Work out the finished part from the listing and answer in its coordinate system (mm). A direction names the side the tool comes from. Give positions to 0.01 mm unless a question says otherwise; leave off trailing zeros. Loops run counter-clockwise (first coordinate to the right, second up) from the corner with the lowest first, then second, coordinate; pieces in that order, holes last. Notation, with made-up numbers: M -17.5,81 L -7.5,81 A25 ccw -7.5,96 Z; hole C 15,31 d1. An arc over 180 degrees is marked long. Write item = value, one per line. Start each with the question number.
1. Section C-C on x = 9 is taken. Determine the outline of the cut face in (y, z).
2. Section D-D on y = 4 is taken. Give the number of separate pieces and of enclosed holes in the cut face, plus the area to 3 significant figures.
3. Flat-ended cylindrical pins translate along their axes: pin 1 Ø12 at (y, z) = (-11.5, 3.5) entering from -X; pin 2 Ø17 at (y, z) = (-7.5, 8) entering from +X; pin 3 Ø8 at (x, y) = (-22, -8.75) entering from -Z. Find the tip coordinate at first contact, or state that the pin passes through.
4. The mould has two halves that part along X. Classify faces 4 (the face through (-13, 0, 13)), 5 (the face through (10.5, -0.3, 17)), 6 (the face through (27, 15, 18)): released by +X, released by -X, zero draft, split by the parting line, or undercut.
5. Consider L1, parallel to Y at x = -22, z = 18; L2, parallel to X at y = 16, z = 14; L3, parallel to Z at x = -6, y = -16. Determine where each line is inside the solid, lowest interval first. Write a range as [from, to].
6. Section B-B on z = 7.5 is taken. Determine the outline of the cut face in (x, y).
7. For faces 1 (the face through (16, 0, -17)), 2 (the face through (48, 0, 17)), 3 (the face through (16.5, 0, -18)), determine the directions among +Z, -Z, +X, -X, +Y, -Y from which every point of the face is accessible in a straight line to the end or side of a thin tool.
8. Section A-A on x = 48.5 is taken. Determine the outline of the cut face in (y, z).
```python
from build123d import *

# Parameters (mm, degrees)
F0_W          = 24
F0_H          = 34
F1_DEPTH      = 18.75
F1_DEPTH_BACK = 18.75
F2_R          = 2.5
F3_DEPTH      = 2.5
F2_W          = 6.75
F2_H          = 30
F2_W_2        = 13.25
F4_DEPTH      = 60
F5_W          = 29.5
F5_H          = 28.5
F6_DEPTH      = 76.15809
F6_DEPTH_BACK = 25


with BuildPart() as f1:
    # F0 (on Front) → F1 (new body, two sides)
    with BuildSketch(Plane.XZ) as f1_sk:
        Polygon((14.5, 19.5), (-14.5, 19.5), (-14.5, -19.5), (14.5, -19.5), (41, -19.5), (41, -17), (41, 17), (41, 19.5), align=None)
        Rectangle(F0_W, F0_H, mode=Mode.SUBTRACT)
        with Locations((26.5, 0)):
            Rectangle(F0_W, F0_H, mode=Mode.SUBTRACT)
    extrude(amount=F1_DEPTH)
    extrude(f1_sk.sketch, amount=-F1_DEPTH_BACK)

    # F2 (on face) → F3 (join)
    with BuildSketch(Plane.XY.offset(19.5)):
        Polygon((-29.5, 18.75), (-29.5, -18.75), (56, -18.75), (56, 18.75), (-14.5, 18.75), align=None)
        with Locations((-22, -8.75)):
            Circle(F2_R, mode=Mode.SUBTRACT)
        with Locations((48.5, -8.75)):
            Circle(F2_R, mode=Mode.SUBTRACT)
        with Locations((-22, 8.75)):
            Circle(F2_R, mode=Mode.SUBTRACT)
        Polygon((-10, -15), (-10, 15), (3.25, 15), (10, 15), (16.5, 15), (23.25, 15), (36.5, 15), (36.5, -15), (23.25, -15), (16.5, -15), (10, -15), (3.25, -15), align=None, mode=Mode.SUBTRACT)
        with Locations((48.5, 8.75)):
            Circle(F2_R, mode=Mode.SUBTRACT)
    extrude(amount=-F3_DEPTH)

    # F2 (on face) → F4 (cut)
    with BuildSketch(Plane.XY.offset(19.5)):
        with Locations((6.625, 0)):
            Rectangle(F2_W, F2_H)
        with Locations((-3.375, 0)):
            Rectangle(F2_W_2, F2_H)
        with Locations((19.875, 0)):
            Rectangle(F2_W, F2_H)
        with Locations((29.875, 0)):
            Rectangle(F2_W_2, F2_H)
    extrude(amount=-F4_DEPTH, mode=Mode.SUBTRACT)

    # F5 (on Right) → F6 (cut, two sides)
    with BuildSketch(Plane.YZ) as f6_sk:
        with Locations((0, -1.25)):
            Rectangle(F5_W, F5_H)
    extrude(amount=F6_DEPTH, mode=Mode.SUBTRACT)
    extrude(f6_sk.sketch, amount=-F6_DEPTH_BACK, mode=Mode.SUBTRACT)


solid = f1.part
```
Verdict:
q1.outline = M -18.75,-19.5 L -15,-19.5 L -15,-17 L -18.75,-17 Z; M -18.75,17 L -15,17 L -15,19.5 L -18.75,19.5 Z; M 15,-19.5 L 18.75,-19.5 L 18.75,-17 L 15,-17 Z; M 15,17 L 18.75,17 L 18.75,19.5 L 15,19.5 Z
q2.separate_pieces = 6
q2.enclosed_holes = 0
q2.area = 194 mm2
q3.pin_1 = -14.5
q3.pin_2 = 41
q3.pin_3 = 17
q4.face_4 = zero draft
q4.face_5 = undercut
q4.face_6 = undercut
q5.L1 = [-18.75, -11.25], [-6.25, 6.25], [11.25, 18.75]
q5.L2 = [-14.5, -12], [12, 14.5], [38.5, 41]
q5.L3 = [-19.5, -17], [17, 19.5]
q6.outline = M -14.5,-18.75 L -12,-18.75 L -12,-14.75 L -14.5,-14.75 Z; M -14.5,14.75 L -12,14.75 L -12,18.75 L -14.5,18.75 Z; M 12,-18.75 L 14.5,-18.75 L 14.5,-14.75 L 12,-14.75 Z; M 12,14.75 L 14.5,14.75 L 14.5,18.75 L 12,18.75 Z; M 38.5,-18.75 L 41,-18.75 L 41,-14.75 L 38.5,-14.75 Z; M 38.5,14.75 L 41,14.75 L 41,18.75 L 38.5,18.75 Z
q7.face_1 = +Y, -Y
q7.face_2 = -Z, +X, +Y, -Y
q7.face_3 = +Z, -Z
q8.outline = M -18.75,17 L -11.25,17 L -11.25,19.5 L -18.75,19.5 Z; M -6.25,17 L 6.25,17 L 6.25,19.5 L -6.25,19.5 Z; M 11.25,17 L 18.75,17 L 18.75,19.5 L 11.25,19.5 Z
